Part print with two shaded views. Sizes in mm from the minimum x, y, z corner. A direction names the side the tool comes from. Round coordinates to 2 decimals unless told otherwise and drop trailing zeros. Loops run counter-clockwise (first coordinate to the right, second up) from the corner with the lowest first, then second, coordinate; pieces in that order, holes last. Notation, with made-up numbers: (5.5, -33) - (22.5, -33) arc R25 cw to (22.5, -21) - close; hole circle Ø6 at (22.25, -20). An arc over 180 degrees is marked (long way). Use a Markdown table: item, result.
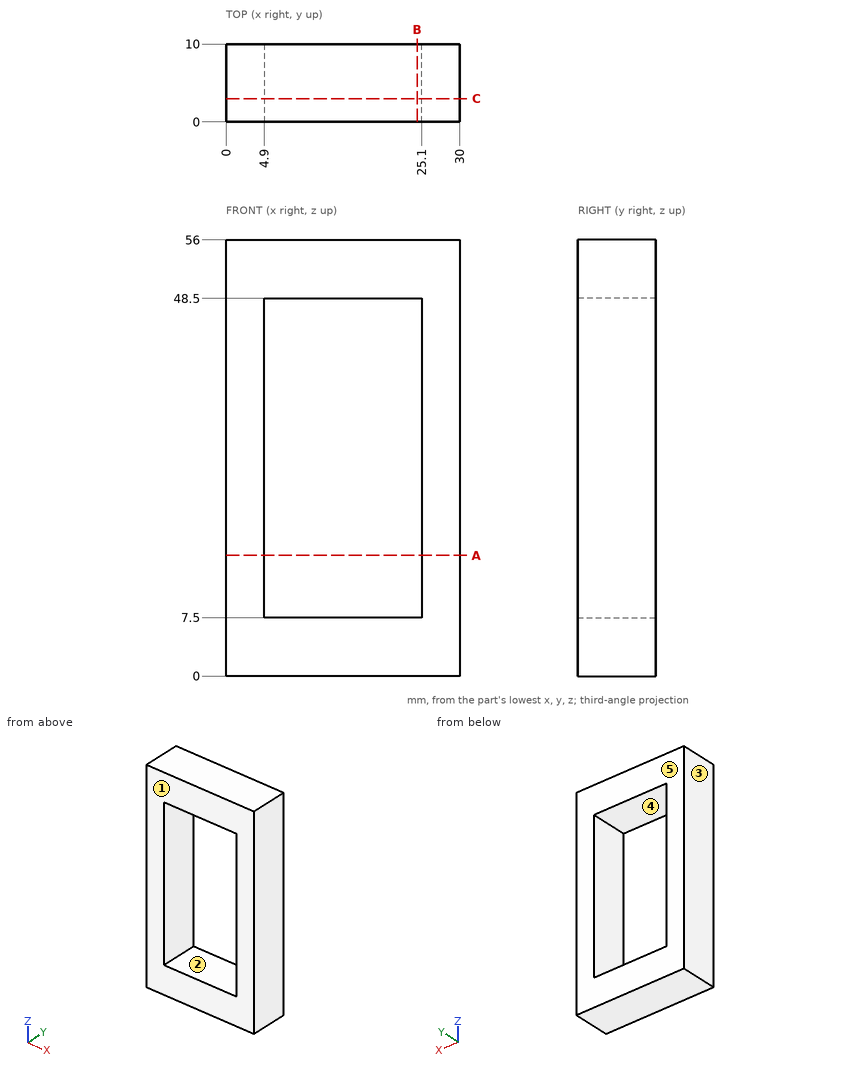
Q1. Drop a flat-ended pin along its axis: pin 1 (10 mm diameter, centred on x = 23, z = 40.5, fed in from +Y). Give the stop position or say it passes through.
Results found:
| item | result |
|---|---|
| pin 1 | stops at y = 10 |
Q2. Which spindle directions (+Z, -Z, +X, -X, +Y, -Y) get a long thin tool onto all of the face, cutting with end or side? Do the marked faces 1 and 2. Say none if no direction does.
Results found:
| item | result |
|---|---|
| face 1 | +Z, -Z, +X, -X, -Y |
| face 2 | +Y, -Y |
Q3. Cut at C-C, the plane y = 3. List the corners of the cut face in (x, z), plus the area to 3 significant figures.
Results found:
| item | result |
|---|---|
| outline | (0, 0) - (30, 0) - (30, 56) - (0, 56) - close; hole (4.9, 7.5) - (25.1, 7.5) - (25.1, 48.5) - (4.9, 48.5) - close |
| area | 852 mm2 |
Q4. Cut at A-A, the plane z = 15.5. List the corners of the cut face in (x, y).
Results found:
| item | result |
|---|---|
| outline | (0, 0) - (4.9, 0) - (4.9, 10) - (0, 10) - close; (25.1, 0) - (30, 0) - (30, 10) - (25.1, 10) - close |
Q5. Probe line 1 (X direction, y = 1.75, z = 39); line 2 (Z direction, x = 21, y = 2.25). List the from-to ranges inside material, lowest first.
Results found:
| item | result |
|---|---|
| line 1 | x = 0 to 4.9, 25.1 to 30 |
| line 2 | z = 0 to 7.5, 48.5 to 56 |
Q6. Cut at B-B, the plane x = 24.5. List the corners of the cut face in (y, z).
Results found:
| item | result |
|---|---|
| outline | (0, 0) - (10, 0) - (10, 7.5) - (0, 7.5) - close; (0, 48.5) - (10, 48.5) - (10, 56) - (0, 56) - close |
Q7. Pull direction X, two halves, no side cores. Call the marked faces 3, 4 and 5: pulls with the +X half, pulls with the -X half, needs draft (parallel to the pull), parting line crosses it, or undercut.
Results found:
| item | result |
|---|---|
| face 3 | pulls with the -X half |
| face 4 | undercut |
| face 5 | needs draft |
